Here's how the part is built. I have some questions about the finished solid (model axes, mm). A direction names the side the tool comes from. Coordinates: 2 decimals unless noted, no trailing zeros. Loops run counter-clockwise (first coordinate to the right, second up) from the corner with the lowest first, then second, coordinate; pieces in that order, holes last. Notation, with made-up numbers: M 35.25,36 L 42.25,36 A29 cw 42.25,70 Z; hole C 37,42 d7. An arc over 180 degrees is marked long. Use CSV: the item, a comma, the result in double quotes. Start each with the question number.
Q1. If we mould it in two halves opening along X, with no side actions, what happens to faces 4 (the flat face through (-15, -6, 1.65)), 5 (the flat face through (-66.277, -51.53, 0.173)), 6 (the cylindrical face through (-27.63, 20.42, 1.32))? For each: +X half, -X half, draft (parallel to the pull), parting line (faces both ways), or undercut.
Q2. Which directions (+Z, -Z, +X, -X, +Y, -Y) give clear straight access to the entire face, cutting with the end or side of a thin tool? Please do faces 1 (the flat face through (-18, 10, 0.35)), 2 (the flat face through (-27, 8, 1.65)), 3 (the cylindrical face through (-31.61, 12.06, 1.32)).
Q3. If we section it at A-A (y = 57): Please give me the cut outline in (x, z), and give its area (3 significant figures).
Q4. If we section it at D-D (y = -45.5): Please give me the cut outline in (x, z), and give its area (3 significant figures).
Q5. If we section it at C-C (x = -4): State how many separate pieces and enclosed holes the cut face has, and give its area (3 significant figures).
Q6. If we section it at B-B (z = 0.95): Please give me the cut outline in (x, y), and give its area (3 significant figures).
Q7. Please list where these lines run through material, in increasing order: probe 1 along Z at (x, y) = (-72, 56.5); probe 2 along Y at (x, z) = (-19, 0.4); probe 3 along Y at (x, z) = (-21.5, 0.6). Write a range as [from, to].
from build123d import *

# Parameters (mm, degrees)
F1_DEPTH = 0.35
F3_DEPTH = 2
F5_DEPTH = 1.3
F6_R     = 1.1


with BuildPart() as f1:
    # F0 (on Top) → F1 (new body)
    with BuildSketch(Plane.XY):
        with BuildLine():
            Line((47.8413986466, -33.0526276553), (47.8413986466, 85.9473723447))
            ThreePointArc((47.8413986466, 85.9473723447), (47.5485054278, 86.6544791259), (46.8413986466, 86.9473723447))
            Line((46.8413986466, 86.9473723447), (-81.1586013534, 86.9473723447))
            ThreePointArc((-81.1586013534, 86.9473723447), (-81.8657081346, 86.6544791259), (-82.1586013534, 85.9473723447))
            Line((-82.1586013534, 85.9473723447), (-82.1586013534, -33.0526276553))
            ThreePointArc((-82.1586013534, -33.0526276553), (-81.7948777262, -34.9247765264), (-80.7566247951, -36.5245474862))
            Line((-80.7566247951, -36.5245474862), (-51.3861264072, -66.9618118353))
            ThreePointArc((-51.3861264072, -66.9618118353), (-49.742636266, -68.0920436291), (-47.7881029655, -68.4898920043))
            Line((-47.7881029655, -68.4898920043), (13.4709002587, -68.4898920043))
            ThreePointArc((13.4709002587, -68.4898920043), (15.4254335591, -68.0920436291), (17.0689237004, -66.9618118353))
            Line((17.0689237004, -66.9618118353), (46.4394220883, -36.5245474862))
            ThreePointArc((46.4394220883, -36.5245474862), (47.4776750193, -34.9247765264), (47.8413986466, -33.0526276553))
        make_face()
        with BuildLine():
            ThreePointArc((-39.1047286936, 78.250517656), (-38.8118354748, 78.9576244372), (-38.1047286936, 79.250517656))
            Line((-38.1047286936, 79.250517656), (4.0952713064, 79.250517656))
            ThreePointArc((4.0952713064, 79.250517656), (4.8023780876, 78.9576244372), (5.0952713064, 78.250517656))
            Line((5.0952713064, 78.250517656), (5.0952713064, 71.050517656))
            ThreePointArc((5.0952713064, 71.050517656), (7.1952713064, 68.950517656), (5.0952713064, 66.850517656))
            Line((5.0952713064, 66.850517656), (5.0952713064, 54.950517656))
            ThreePointArc((5.0952713064, 54.950517656), (4.8023780876, 54.2434108748), (4.0952713064, 53.950517656))
            Line((4.0952713064, 53.950517656), (-38.1047286936, 53.950517656))
            ThreePointArc((-38.1047286936, 53.950517656), (-38.8118354748, 54.2434108748), (-39.1047286936, 54.950517656))
            Line((-39.1047286936, 54.950517656), (-39.1047286936, 66.850517656))
            ThreePointArc((-39.1047286936, 66.850517656), (-41.2047286936, 68.950517656), (-39.1047286936, 71.050517656))
            Line((-39.1047286936, 71.050517656), (-39.1047286936, 78.250517656))
        make_face(mode=Mode.SUBTRACT)
    extrude(amount=F1_DEPTH)

    # F2 (on face) → F3 (cut)
    with BuildSketch(Plane.XY.offset(0.35)):
        Polygon((13.2559401929, -49.3898926318), (-30.2440598071, -49.3898926318), (-30.2440598071, -53.7898926318), (-38.2440598071, -53.7898926318), (-38.2440598071, -59.7898926318), (-30.2440598071, -59.7898926318), (13.2559401929, -59.7898926318), align=None)
    extrude(amount=-F3_DEPTH, mode=Mode.SUBTRACT)

    # F4 (on face) → F5 (join)
    with BuildSketch(Plane.XY.offset(0.35)):
        Polygon((-35.7913524045, 35.1850536081), (-28.1538574591, -10.5309743335), (-18.6824351945, 5.5515397377), align=None)
        Polygon((18.5652113225, 7.5971377061), (-24.9834829413, 23.4652745761), (-15.6513462812, 7.3015397377), align=None)
        Polygon((-33.1309387548, -25.878880379), (3.1361268654, 3.9696324182), (-15.6513462812, 3.8015397377), align=None)
    extrude(amount=F5_DEPTH)

    # F6
    f6_edges = [f1.edges().sort_by_distance(p)[0] for p in [
        (-14.997406, -10.954624, 1.65),
        (-6.25761, 3.885586, 1.65),
        (-24.391143, -11.03867, 1.65),
        (-31.972605, 12.32704, 1.65),
        (-23.418146, -2.489717, 1.65),
        (-27.236894, 20.368297, 1.65),
        (1.456933, 7.449339, 1.65),
        (-3.209136, 15.531206, 1.65),
        (-20.317415, 15.383407, 1.65),
    ]]
    fillet(f6_edges, radius=F6_R)


solid = f1.part
Results below:
1,face 4,"draft"
1,face 5,"-X half"
1,face 6,"undercut"
2,face 1,"+Z"
2,face 2,"+Z, +X, -X, +Y, -Y"
2,face 3,"+Z, -X"
3,outline,"M -82.16,0 L -39.1,0 L -39.1,0.35 L -82.16,0.35 Z; M 5.1,0 L 47.84,0 L 47.84,0.35 L 5.1,0.35 Z"
3,area,"30.0 mm^2"
4,outline,"M -72.1,0 L 37.78,0 L 37.78,0.35 L -72.1,0.35 Z"
4,area,"38.5 mm^2"
5,separate pieces,"3"
5,enclosed holes,"0"
5,area,"59.3 mm^2"
6,outline,"M -35.65,34.79 L -28.11,-10.31 L -18.77,5.55 Z; M -32.85,-25.55 L 2.92,3.89 L -15.61,3.73 Z; M -24.81,23.32 L -15.61,7.38 L 18.15,7.67 Z"
6,area,"811 mm^2"
7,probe 1,"[0, 0.35]"
7,probe 2,"[-14.25, -1.88], [5.01, 6.1], [13.1, 21.29]"
7,probe 3,"[-16.3, -6.13], [0.77, 10.43], [17.43, 22.19]"
